The figure shows three views and two pictorial views of one solid part (mm, origin at its lowest corner). Answer the questions. A direction names the side the tool comes from. Round coordinates to 2 decimals unless told otherwise and drop trailing zeros. Order: outer loops, then holes, each group sorted by start corner. A loop starts at its lowest first (then second) coordinate and runs counter-clockwise, first axis right, second up. Notation, with made-up numbers: (-25, 66.25) - (31, 66.25) arc R33 cw to (31, 95.25) - close; hole circle Ø3 at (78.5, -9.75). An arc over 180 degrees is marked (long way). Answer in a Markdown table with one row per item.
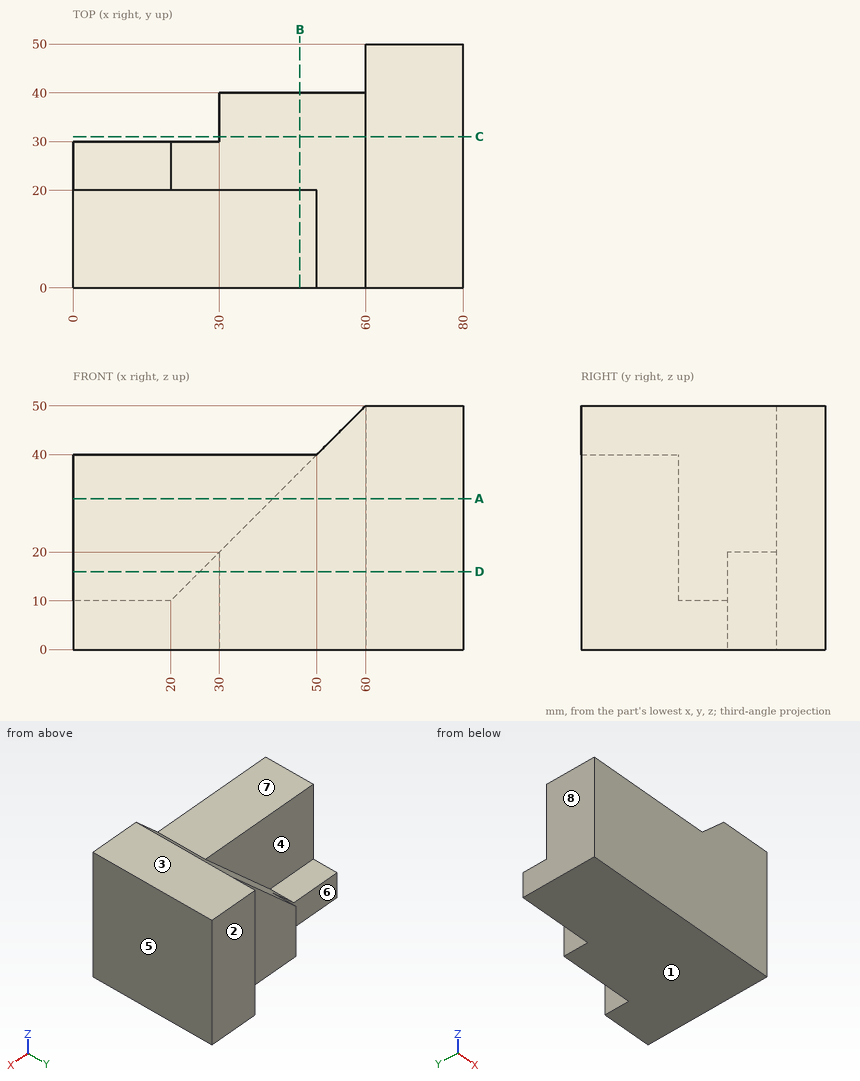
1) Each of these flat-tipped pins is pushed along its axis until it touches: pin 1 (16 mm diameter, centred on x = 16, z = 10.5, fed in from +Y); pin 2 (8 mm diameter, centred on x = 38, y = 6, fed in from +Z); pin 3 (8 mm diameter, centred on y = 45.5, z = 19.5, fed in from -X). Where does it stop, or does it pass through?
Filled in:
| item | result |
|---|---|
| pin 1 | stops at y = 30 |
| pin 2 | stops at z = 40 |
| pin 3 | stops at x = 60 |
2) Which of the six approach directions +Z, -Z, +X, -X, +Y, -Y give full straight-line access (tool end or side, diameter ignored) to the marked faces 4, 5, 6, 7 and 8?
Filled in:
| item | result |
|---|---|
| face 4 | +Z, -X, +Y |
| face 5 | +Z, -Z, +X, +Y, -Y |
| face 6 | +Z, -Z, -X, +Y |
| face 7 | +Z, -X, +Y, -Y |
| face 8 | +Z, -Z, -X, +Y, -Y |
3) Find the intervals of material crossed by probe 1 along Z at (x, y) = (40, 19.5); probe 2 along X at (y, z) = (36, 17); probe 3 along X at (y, z) = (41, 42.5), in increasing order. Write a range as from..to.
Filled in:
| item | result |
|---|---|
| probe 1 | z = 0..40 |
| probe 2 | x = 30..80 |
| probe 3 | x = 60..80 |
4) Find section B-B, the plane x = 46.5. Give the vertices of the cut face in (y, z), then the cut area to 3 significant figures.
Filled in:
| item | result |
|---|---|
| outline | (0, 0) - (40, 0) - (40, 36.5) - (20, 36.5) - (20, 40) - (0, 40) - close |
| area | 1,530 mm^2 |
5) Find section A-A, the plane z = 31. Give the vertices of the cut face in (x, y).
Filled in:
| item | result |
|---|---|
| outline | (0, 0) - (80, 0) - (80, 50) - (60, 50) - (60, 40) - (41, 40) - (41, 20) - (0, 20) - close |
6) Find section C-C, the plane y = 31. Give the vertices of the cut face in (x, z), then the cut area to 3 significant figures.
Filled in:
| item | result |
|---|---|
| outline | (30, 0) - (80, 0) - (80, 50) - (60, 50) - (30, 20) - close |
| area | 2,050 mm^2 |
7) Find section D-D, the plane z = 16. Give the vertices of the cut face in (x, y).
Filled in:
| item | result |
|---|---|
| outline | (0, 0) - (80, 0) - (80, 50) - (60, 50) - (60, 40) - (30, 40) - (30, 30) - (26, 30) - (26, 20) - (0, 20) - close |
8) The mould has two halves that part along Z. Classify the marked faces 1, 2 and 3: released by +Z, released by -Z, zero draft, split by the parting line, or undercut.
Filled in:
| item | result |
|---|---|
| face 1 | released by -Z |
| face 2 | zero draft |
| face 3 | released by +Z |
